Verification items for the finished model (mm, model axes). Face numbers are marked on the shaded views. A direction names the side the tool comes from. Round coordinates to 2 decimals unless told otherwise and drop trailing zeros. Write each loop counter-clockwise with the first axis right and the second up, starting at its lowest first coordinate (ties: lowest second). Pieces come first, ordered by that corner, then holes. Notation, with made-up numbers: M 3,77 L 50,77 A20 cw 50,93 Z; hole C 33.25,8 d7. An arc over 180 degrees is marked long. One line per item, written item: value. Start each with the question number.
Item 1: Section check A-A, the plane y = -8. Record the cut outline in (x, z), then the cut area to 3 significant figures.
Item 2: Draft check along X on the marked faces 1, 2, 3 and 4. Enter one of: +X half, -X half, draft (parallel to the pull), parting line (faces both ways), or undercut.
Item 3: Section check C-C, the plane x = 25. Record the cut outline in (y, z), then the cut area to 3 significant figures.
Item 4: Gauge pin test, flat ends, axial feed: pin 1 (5 mm diameter, centred on y = -1.5, z = -4, fed in from -X); pin 2 (5 mm diameter, centred on y = 0, z = -5.5, fed in from +X); pin 3 (2 mm diameter, centred on x = -3.24, y = -8, fed in from +Z); pin 4 (12 mm diameter, centred on x = -7.5, y = 3.5, fed in from -Z). Record the tip position at first contact, or that the pin passes through.
Item 5: Tool access check on the marked faces 5, 6, 7, 8 and 9. Record the directions out of +Z, -Z, +X, -X, +Y, -Y that give a thin tool (end or side, any length) a straight path to the whole face; none if there is none.
Item 6: Section check B-B, the plane z = -7.5. Record the cut outline in (x, y).
Item 7: Thickness scan on probe 1 along X at (y, z) = (-1.5, -1); probe 2 along X at (y, z) = (-1, -6.75); probe 3 along Y at (x, z) = (-11.5, -11.25). Record the ranges inside material, lowest first. Write a range as from..to.
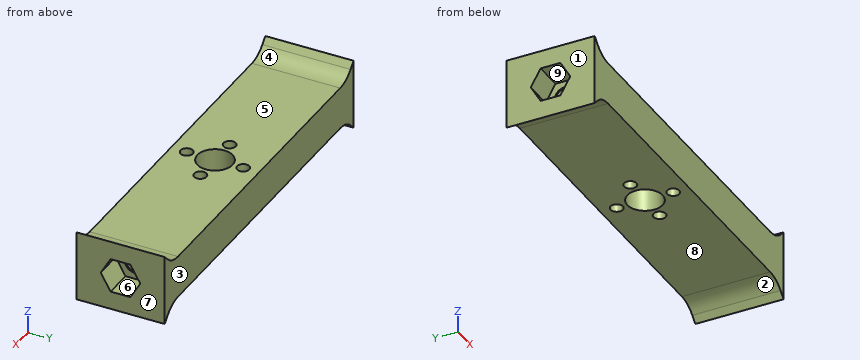
Solid Edge part; units mm, degrees
sketch "Sketch1" plane through (0, 0, 0) normal (0, 0, 1) x (1, 0, 0)
  line L0 (48.2617, 12.5) -> (-54.7383, 12.5)
  line L1 (-54.7383, 12.5) -> (-54.7383, -12.5)
  line L2 (-54.7383, -12.5) -> (48.2617, -12.5)
  line L3 (48.2617, -12.5) -> (48.2617, 12.5)
  circle A0 centre (-11.2383, 0) radius 1.75
  circle A1 centre (-3.2383, -8) radius 1.75
  circle A2 centre (4.7617, 0) radius 1.75
  circle A3 centre (-3.2383, 0) radius 5
  circle A4 centre (-3.2383, 8) radius 1.75
extrude "Protrusion1" add sketch "Sketch1" against normal blind 12
sketch "Sketch2" plane through (-54.7383, 0, -6) normal (-1, 0, 0) x (0, 0, -1)
  line L0 (4.85, 2.8001) -> (0, 5.6003)
  line L1 (0, 5.6003) -> (-4.85, 2.8001)
  line L2 (-4.85, 2.8001) -> (-4.85, -2.8001)
  line L3 (-4.85, -2.8001) -> (0, -5.6003)
  line L4 (0, -5.6003) -> (4.85, -2.8001)
  line L5 (4.85, -2.8001) -> (4.85, 2.8001)
extrude "ExtrudedCutout_2" cut sketch "Sketch2" against normal blind 8.1
sketch "Sketch3" plane through (48.2617, 0, -6) normal (1, 0, 0) x (0, 0, 1)
  line L0 (4.85, 2.8001) -> (0, 5.6003)
  line L1 (0, 5.6003) -> (-4.85, 2.8001)
  line L2 (-4.85, 2.8001) -> (-4.85, -2.8001)
  line L3 (-4.85, -2.8001) -> (0, -5.6003)
  line L4 (0, -5.6003) -> (4.85, -2.8001)
  line L5 (4.85, -2.8001) -> (4.85, 2.8001)
extrude "ExtrudedCutout_3" cut sketch "Sketch3" against normal blind 8.1
sketch "Sketch4" plane through (-4.7383, -12.5, -6) normal (0, -1, 0) x (-1, 0, 0)
  line L0 (-53, 10) -> (-49, 6)
  line L1 (-53, 6) -> (-49, 6)
  line L2 (-53, 6) -> (-53, 10)
  line L3 (-53, -6) -> (-53, -10)
  line L4 (-53, -10) -> (-49, -6)
  line L5 (-53, -6) -> (-49, -6)
  line L6 (50, 10) -> (46, 6)
  line L7 (46, 6) -> (50, 6)
  line L8 (50, 6) -> (50, 10)
  line L9 (50, -10) -> (46, -6)
  line L10 (50, -6) -> (46, -6)
  line L11 (50, -6) -> (50, -10)
extrude "ExtrudedProtrusion_8" add sketch "Sketch4" against normal blind 25
sketch "Sketch5" plane through (40.1617, 0, -6) normal (1, 0, 0) x (0, -0.5, 0.866)
  circle A0 centre (0, 0) radius 3.15
extrude "ExtrudedCutout_4" cut sketch "Sketch5" against normal blind 0.5
sketch "Sketch6" plane through (-46.6383, 0, -6) normal (-1, 0, 0) x (0, 0.5, -0.866)
  circle A0 centre (0, 0) radius 3.15
extrude "ExtrudedCutout_5" cut sketch "Sketch6" against normal blind 0.5
fillet "Round_2" radius 8 4 edges at (44.2617, 0, 0) (44.2617, 0, -12) (-50.7383, 0, -12) (-50.7383, 0, 0)
Response values:
1. outline: M -54.74,-16 L -53.08,-14.34 A8 cw -47.42,-12 L -4.99,-12 L -4.99,0 L -47.42,0 A8 cw -53.08,2.34 L -54.74,4 Z; M -1.49,-12 L 40.95,-12 A8 cw 46.6,-14.34 L 48.26,-16 L 48.26,4 L 46.6,2.34 A8 cw 40.95,0 L -1.49,0 Z
1. area: 1,230 mm2
2. face 1: -X half
2. face 2: undercut
2. face 3: draft
2. face 4: undercut
3. outline: M -12.5,-12 L 12.5,-12 L 12.5,0 L -12.5,0 Z
3. area: 300 mm2
4. pin 1: stops at x = -46.64
4. pin 2: stops at x = 39.66
4. pin 3: passes through
4. pin 4: stops at z = -12
5. face 5: +Z, +Y, -Y
5. face 6: +X
5. face 7: +Z, -Z, +X, +Y, -Y
5. face 8: -Z, +Y, -Y
5. face 9: -X
6. outline: M -54.74,-12.5 L 48.26,-12.5 L 48.26,-4.73 L 40.16,-4.73 L 40.16,-2.77 L 39.66,-2.77 L 39.66,2.77 L 40.16,2.77 L 40.16,4.73 L 48.26,4.73 L 48.26,12.5 L -54.74,12.5 L -54.74,4.73 L -46.64,4.73 L -46.64,2.77 L -46.14,2.77 L -46.14,-2.77 L -46.64,-2.77 L -46.64,-4.73 L -54.74,-4.73 Z; hole C -11.24,0 d3.5; hole C -3.24,0 d10; hole C -3.24,-8 d3.5; hole C -3.24,8 d3.5; hole C 4.76,0 d3.5
7. probe 1: x = -54.74..-12.14, -10.34..-8.01, 1.53..3.86, 5.66..48.26
7. probe 2: x = -46.14..-12.67, -9.8..-8.14, 1.66..3.33, 6.2..39.66
7. probe 3: y = -12.5..-1.73, 1.73..12.5
